```python
from build123d import *

# Parameters (mm, degrees)
EXTRUDE_1_DEPTH     = 3
SKETCH_2_R          = 1.1
SKETCH_2_R_2        = 1.025013192
SKETCH_2_R_3        = 1.6
CUT_EXTRUDE_2_DEPTH = 111.535062311
FILLET_1_R          = 5


with BuildPart() as part:
    # 草图1 → 凸台-拉伸1 (new body)
    with BuildSketch(Plane.XY):
        Polygon((0, 0), (0, -47), (-42, -47), (-100, -5), (-100, 0), align=None)
    extrude(amount=EXTRUDE_1_DEPTH)

    # 草图2 → 切除-拉伸2 (cut, through all)
    with BuildSketch(Plane.XY.offset(3)):
        with Locations(Location((-38, -35, 0), (0, 0, 180))):
            Circle(SKETCH_2_R)
        with Locations(Location((-38, -14.5, 0), (0, 0, 180))):
            Circle(SKETCH_2_R)
        with Locations(Location((-38, -2.5, 0), (0, 0, 180))):
            Circle(SKETCH_2_R)
        with Locations(Location((-56, -2.5, 0), (0, 0, 180))):
            Circle(SKETCH_2_R)
        with Locations(Location((-74, -2.5, 0), (0, 0, 180))):
            Circle(SKETCH_2_R)
        with Locations(Location((-92, -2.5, 0), (0, 0, 180))):
            Circle(SKETCH_2_R)
        with Locations((-56.501870582, -34.029333193)):
            Circle(SKETCH_2_R_2)
        with Locations((-69.609581311, -24.853935684)):
            Circle(SKETCH_2_R_2)
        with Locations((-82.717292039, -15.678538174)):
            Circle(SKETCH_2_R_2)
        with Locations((-20, -2.5)):
            Circle(SKETCH_2_R)
        with Locations((-2, -2.5)):
            Circle(SKETCH_2_R)
        with Locations((-2, -14.5)):
            Circle(SKETCH_2_R)
        with Locations((-2, -35)):
            Circle(SKETCH_2_R)
        with Locations((-5, -44)):
            Circle(SKETCH_2_R_3)
        with Locations((-25, -44)):
            Circle(SKETCH_2_R_3)
    extrude(amount=-CUT_EXTRUDE_2_DEPTH, mode=Mode.SUBTRACT)

    # 圆角1
    fillet_1_edges = [part.edges().sort_by_distance(p)[0] for p in [
        (-100, -5, 1.5),
    ]]
    fillet(fillet_1_edges, radius=FILLET_1_R)


solid = part.part
```
Input: part model. Units: mm. Frame: model coordinates. Coordinates: 2 decimals unless noted, no trailing zeros. Order: outer loops, then holes, each group sorted by start corner. A loop starts at its lowest first (then second) coordinate and runs counter-clockwise, first axis right, second up. Notation, with made-up numbers: (10, -40) - (25, -40) arc R17 ccw to (25, -10) - close; hole circle Ø7 at (-19, -26.5). An arc over 180 degrees is marked (long way). Return JSON: item names as keys, results as strings.
Q1. Cut plane A-A (x = -5). Return loops of the section in (y, z).
The answers:
{"outline": "(-47, 0) - (-45.6, 0) - (-45.6, 3) - (-47, 3) - close; (-42.4, 0) - (0, 0) - (0, 3) - (-42.4, 3) - close"}
Q2. Cut plane D-D (z = 2.25). State how many separate pieces and enclosed holes the cut face has, then the cut area to 3 significant figures.
The answers:
{"separate pieces": "1", "enclosed holes": "15", "area": "3,420 mm2"}
Q3. Cut plane B-B (x = -38). Return loops of the section in (y, z).
The answers:
{"outline": "(-47, 0) - (-36.1, 0) - (-36.1, 3) - (-47, 3) - close; (-33.9, 0) - (-15.6, 0) - (-15.6, 3) - (-33.9, 3) - close; (-13.4, 0) - (-3.6, 0) - (-3.6, 3) - (-13.4, 3) - close; (-1.4, 0) - (0, 0) - (0, 3) - (-1.4, 3) - close"}
Q4. First-contact query: pin 1 (2.5 mm diameter, centred on x = -25, y = -44, fed in from -Z). Flat tip, straight axial feed; report the tip coordinate or a pass-through.
The answers:
{"pin 1": "passes through"}
Q5. Cut plane C-C (y = -44). Return loops of the section in (x, z).
The answers:
{"outline": "(-46.14, 0) - (-26.6, 0) - (-26.6, 3) - (-46.14, 3) - close; (-23.4, 0) - (-6.6, 0) - (-6.6, 3) - (-23.4, 3) - close; (-3.4, 0) - (0, 0) - (0, 3) - (-3.4, 3) - close"}
Q6. Draft query along X for faces 1 (the flat face through (-69.575, -27.032, 1.479)), 2 (the flat face through (-38, -18, 0)), 3 (the flat face through (0, -23, 1)), 4 (the cylindrical face through (-72.9, -2.5, 1.5)). Return one class per face: +X half, -X half, draft (parallel to the pull), parting line (faces both ways), or undercut.
The answers:
{"face 1": "-X half", "face 2": "draft", "face 3": "+X half", "face 4": "undercut"}
Q7. Ray query, probe 1 along Y at (x, z) = (-38, 0.75); probe 2 along X at (y, z) = (-34, 0.15); probe 3 along Y at (x, z) = (-5, 1.4). Return the intervals inside material, ascending.
The answers:
{"probe 1": "y = -47 to -36.1, -33.9 to -15.6, -13.4 to -3.6, -1.4 to 0", "probe 2": "x = -59.95 to -57.53, -55.48 to -38.46, -37.54 to -2.46, -1.54 to 0", "probe 3": "y = -47 to -45.6, -42.4 to 0"}
